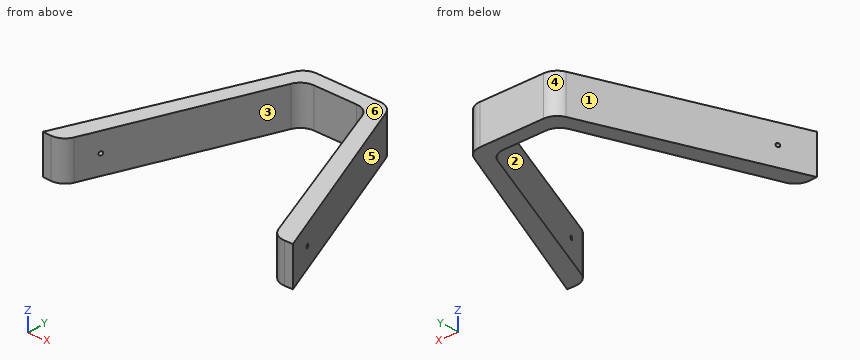
from build123d import *

# Parameters (mm, degrees)
F1_DEPTH      = 12.7
F2_R          = 0.6
F3_DEPTH      = 85.2
F3_DEPTH_BACK = 66
F4_R          = 5


with BuildPart() as f1:
    # F0 (on Top) → F1 (new body)
    with BuildSketch(Plane.XY):
        Polygon((-10.35969, 34.220118), (0, 34.220118), (0, 38.953215), (-13.748372, 38.953215), (-40.783513, -26.551465), (-34.636915, -26.774898), align=None)
        Polygon((0, 38.953215), (0, 34.220118), (10.35969, 34.220118), (34.636915, -26.774898), (40.783513, -26.551465), (13.748372, 38.953215), align=None)
    extrude(amount=F1_DEPTH)

    # F2 (on Right) → F3 (cut, two sides)
    with BuildSketch(Plane.YZ) as f3_sk:
        with Locations((-16.804494, 6.35)):
            Circle(F2_R)
    extrude(amount=F3_DEPTH, mode=Mode.SUBTRACT)
    extrude(f3_sk.sketch, amount=-F3_DEPTH_BACK, mode=Mode.SUBTRACT)

    # F4
    f4_edges = [f1.edges().sort_by_distance(p)[0] for p in [
        (13.748372, 38.953215, 6.35),
        (-13.748372, 38.953215, 6.35),
        (-34.636915, -26.774898, 6.35),
        (34.636915, -26.774898, 6.35),
        (-10.35969, 34.220118, 6.35),
        (10.35969, 34.220118, 6.35),
    ]]
    fillet(f4_edges, radius=F4_R)


solid = f1.part
Source: CAD feature listing. Evaluate the final solid. Frame: model axes, mm. Face numbers are marked on the shaded views. A direction names the side the tool comes from. Round coordinates to 2 decimals unless told otherwise and drop trailing zeros. Order: outer loops, then holes, each group sorted by start corner. A loop starts at its lowest first (then second) coordinate and runs counter-clockwise, first axis right, second up. Notation, with made-up numbers: (66, -2.75) - (94, -2.75) arc R22 ccw to (94, 8.25) - close; hole circle Ø3 at (61.5, 33.25). An arc over 180 degrees is marked (long way). Use a Markdown table: item, result. Add a question column.
1. Section query D-D (x = 4.5). Return the cut outline in (y, z).
2. Set-up query: the marked faces 1 and 2. Return all of +Z, -Z, +X, -X, +Y, -Y with unobstructed straight access to the full face (end or side cutting, diameter ignored); none if empty.
3. Mould query, pull axis X, two halves, no side actions, for the marked faces 3, 4, 5 and 6. Classes: +X half, -X half, draft (parallel to the pull), parting line (faces both ways), or undercut.
4. Line query: probe 1 along Y at (x, z) = (1.5, 11.75); probe 2 along X at (y, z) = (-23.5, 3.75); probe 3 along Y at (x, z) = (34.5, 6.35). Output: solid intervals per line, ascending.
5. Section query C-C (z = 10.25). Return the cut outline in (x, y), then the cut area to 3 significant figures.
6. Section query B-B (y = -15). Return the cut outline in (x, z), then the cut area to 3 significant figures.
7. Section query A-A (x = -35). Return the cut outline in (y, z), then the cut area to 3 significant figures.
8. First-contact query: pin 1 (1.1 mm diameter, centred on y = -16.8, z = 6.35, fed in from -X); pin 2 (3 mm diameter, centred on x = 9, z = 7, fed in from -Y); pin 3 (1.4 mm diameter, centred on y = -16.8, z = 6.35, fed in from +X); pin 4 (3 mm diameter, centred on x = 32.5, z = 4, fed in from -Y). Flat tips, straight axial feed; report the tip coordinate or a pass-through.
Derived:
| question | item | result |
|---|---|---|
| 1 | outline | (34.22, 0) - (38.95, 0) - (38.95, 12.7) - (34.22, 12.7) - close |
| 2 | face 1 | +Z, -Z, -X, +Y |
| 2 | face 2 | +Z, -Z, -Y |
| 3 | face 3 | undercut |
| 3 | face 4 | -X half |
| 3 | face 5 | +X half |
| 3 | face 6 | draft |
| 4 | probe 1 | 34.22 to 38.95 |
| 4 | probe 2 | -39.52 to -33.33, 33.33 to 39.52 |
| 4 | probe 3 | -25.24 to -17.4, -16.2 to -11.33 |
| 5 | outline | (-40.78, -26.55) - (-38.16, -26.65) arc R5 ccw to (-33.33, -23.5) - (-11.61, 31.07) arc R5 cw to (-6.97, 34.22) - (6.97, 34.22) arc R5 cw to (11.61, 31.07) - (33.33, -23.5) arc R5 ccw to (38.16, -26.65) - (40.78, -26.55) - (15.02, 35.86) arc R5 ccw to (10.4, 38.95) - (-10.4, 38.95) arc R5 ccw to (-15.02, 35.86) - close |
| 5 | area | 840 mm2 |
| 6 | outline | (-36.02, 0) - (-29.95, 0) - (-29.95, 12.7) - (-36.02, 12.7) - close; (29.95, 0) - (36.02, 0) - (36.02, 12.7) - (29.95, 12.7) - close |
| 6 | area | 154 mm2 |
| 7 | outline | (-25.67, 0) - (-12.54, 0) - (-12.54, 12.7) - (-25.67, 12.7) - close; hole circle Ø1.2 at (-16.8, 6.35) |
| 7 | area | 166 mm2 |
| 8 | pin 1 | through |
| 8 | pin 2 | y = 32.76 |
| 8 | pin 3 | x = 37.05 |
| 8 | pin 4 | y = -24.68 |
